from build123d import *

# Parameters (mm, degrees)
SKETCH1_R           = 85
SKETCH1_R_2         = 12.5
BOSS_EXTRUDE1_DEPTH = 3
CUT_EXTRUDE1_DEPTH  = 10


with BuildPart() as part:
    # Sketch1 → Boss-Extrude1 (new body)
    with BuildSketch(Plane(origin=(0, 0, 0), x_dir=(1, 0, 0), z_dir=(0, 1, 0))):
        with Locations(Location((0, 0, 0), (0, 0, 270))):
            Circle(SKETCH1_R)
        with Locations(Location((0, 0, 0), (0, 0, 270))):
            Circle(SKETCH1_R_2, mode=Mode.SUBTRACT)
    extrude(amount=BOSS_EXTRUDE1_DEPTH)

    # Sketch2 → Cut-Extrude1 (cut)
    with BuildSketch(Plane(origin=(0, 3, 0), x_dir=(1, 0, 0), z_dir=(0, 1, 0))):
        with BuildLine():
            ThreePointArc((-14, 15.5), (-16.560660172, 16.560660172), (-15.5, 14))
            Line((-15.5, 14), (-15.5, 15.5))
            Line((-15.5, 15.5), (-14, 15.5))
        make_face()
        with BuildLine():
            Line((-15.5, 15.5), (-15.5, 14))
            ThreePointArc((-15.5, 14), (-14.439339828, 14.439339828), (-14, 15.5))
            Line((-14, 15.5), (-15.5, 15.5))
        make_face()
        with BuildLine():
            ThreePointArc((14, 15.5), (14.439339828, 14.439339828), (15.5, 14))
            Line((15.5, 14), (15.5, 15.5))
            Line((15.5, 15.5), (14, 15.5))
        make_face()
        with BuildLine():
            Line((15.5, 15.5), (15.5, 14))
            ThreePointArc((15.5, 14), (16.560660172, 14.439339828), (17, 15.5))
            ThreePointArc((17, 15.5), (15.5, 17), (14, 15.5))
            Line((14, 15.5), (15.5, 15.5))
        make_face()
        with BuildLine():
            ThreePointArc((15.5, -14), (14.439339828, -14.439339828), (14, -15.5))
            Line((14, -15.5), (15.5, -15.5))
            Line((15.5, -15.5), (15.5, -14))
        make_face()
        with BuildLine():
            Line((15.5, -15.5), (14, -15.5))
            ThreePointArc((14, -15.5), (15.5, -17), (17, -15.5))
            ThreePointArc((17, -15.5), (16.560660172, -14.439339828), (15.5, -14))
            Line((15.5, -14), (15.5, -15.5))
        make_face()
        with BuildLine():
            Line((-15.5, -14), (-15.5, -15.5))
            Line((-15.5, -15.5), (-14, -15.5))
            ThreePointArc((-14, -15.5), (-14.439339828, -14.439339828), (-15.5, -14))
        make_face()
        with BuildLine():
            Line((-14, -15.5), (-15.5, -15.5))
            Line((-15.5, -15.5), (-15.5, -14))
            ThreePointArc((-15.5, -14), (-16.560660172, -16.560660172), (-14, -15.5))
        make_face()
    extrude(amount=-CUT_EXTRUDE1_DEPTH, mode=Mode.SUBTRACT)


solid = part.part
Verification items for the finished model (mm, model axes). Coordinates: 2 decimals unless noted, no trailing zeros. Write each loop counter-clockwise with the first axis right and the second up, starting at its lowest first coordinate (ties: lowest second). Pieces come first, ordered by that corner, then holes. Notation, with made-up numbers: M 41,74.25 L 52,74.25 A33 cw 52,105.25 Z; hole C -6,-33 d1. An arc over 180 degrees is marked long. Use CSV: the item, a comma, the result in double quotes.
Q1. Section check C-C, the plane z = 0. Enter the section's corners in (x, y), and give its area (3 significant figures).
Computed values:
outline,"M -85,0 L -12.5,0 L -12.5,3 L -85,3 Z; M 12.5,0 L 85,0 L 85,3 L 12.5,3 Z"
area,"435 mm²"
Q2. Section check B-B, the plane x = 0. Enter the section's corners in (y, z), and give its area (3 significant figures).
Computed values:
outline,"M 0,-85 L 3,-85 L 3,-12.5 L 0,-12.5 Z; M 0,12.5 L 3,12.5 L 3,85 L 0,85 Z"
area,"435 mm²"
Q3. Section check D-D, the plane x = 73. Enter the section's corners in (y, z).
Computed values:
outline,"M 0,-43.54 L 3,-43.54 L 3,43.54 L 0,43.54 Z"
Q4. Go/stop test with flat-tipped pins: P1, Ø1.5, axis at y = 1, z = -19.5, coming from the +X side; P2, Ø1, axis at y = 1, z = 38.5, coming from the +X side. Record where each tip stops, or that it passes through.
Computed values:
P1,"x = 82.91"
P2,"x = 76.03"
Q5. Mould release check, pull along X, two halves, no side actions. Record for faces 1 (the cylindrical face through (-51.721, 1.479, -67.453)), 2 (the cylindrical face through (3.755, 1.479, 11.923)), 3 (the flat face through (-18, 0, -1)): pulls with the +X half, pulls with the -X half, needs draft (parallel to the pull), parting line crosses it, or undercut.
Computed values:
face 1,"parting line crosses it"
face 2,"undercut"
face 3,"needs draft"
Q6. Section check A-A, the plane y = 1.95. Enter the section's corners in (x, z), and give its area (3 significant figures).
Computed values:
outline,"C 0,0 d170; hole C -15.5,-15.5 d3; hole C -15.5,15.5 d3; hole C 0,0 d25; hole C 15.5,-15.5 d3; hole C 15.5,15.5 d3"
area,"22,200 mm²"
Q7. Thickness scan on line 1 along X through (y, z) = (1.1, -15.5); line 2 along X through (y, z) = (1.7, 0). Record the ranges inside material, lowest first. Write a range as [from, to].
Computed values:
line 1,"[-83.57, -17], [-14, 14], [17, 83.57]"
line 2,"[-85, -12.5], [12.5, 85]"
